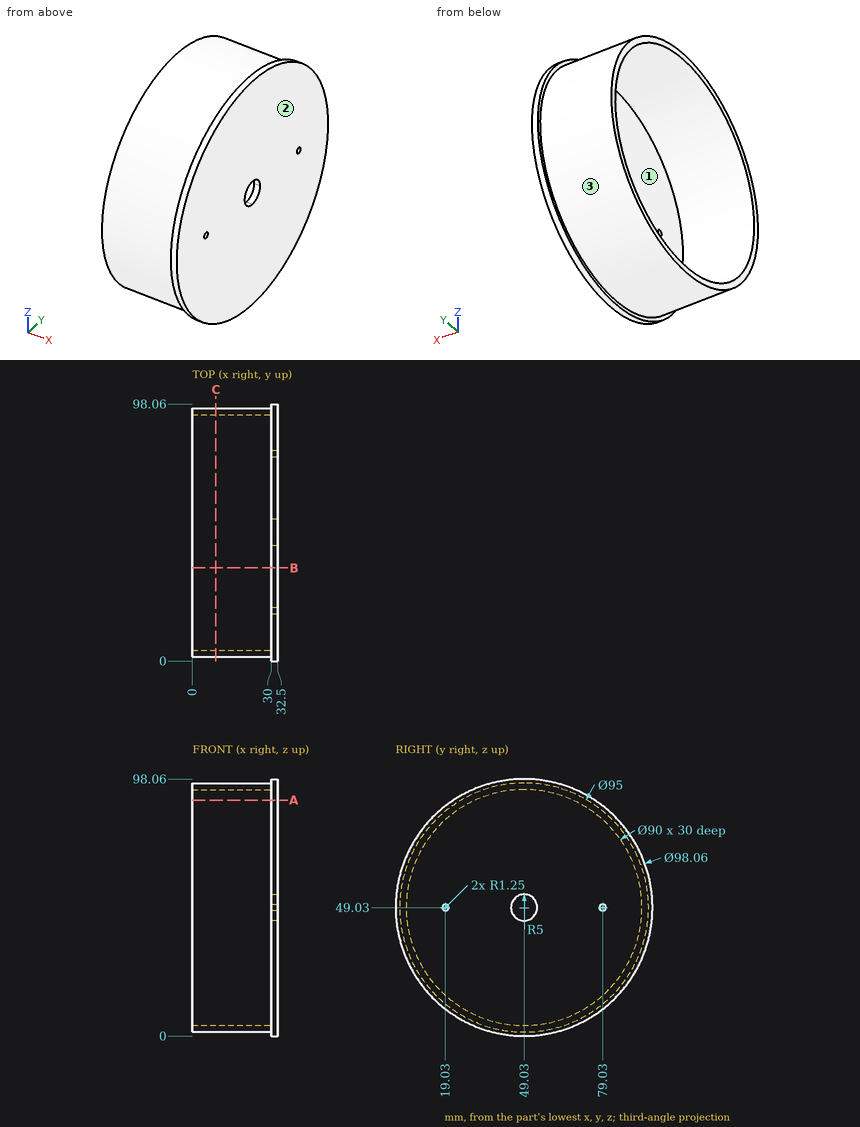
Check sheet for the drawn part. Datum: minimum x, y, z corner. Units: mm. Round coordinates to 2 decimals unless told otherwise and drop trailing zeros. Order: outer loops, then holes, each group sorted by start corner. A loop starts at its lowest first (then second) coordinate and runs counter-clockwise, first axis right, second up. Notation, with made-up numbers: (74.5, 32.5) -> (130.5, 32.5) arc R34 ccw to (130.5, 65.5) -> close; hole circle Ø4 at (61, 42.5). An arc over 180 degrees is marked (long way). Return JSON: item names as keys, results as strings. Group by question number.
Q1. Section check A-A, the plane z = 90. Record the boundary of the cut face in (x, y).
Q2. Section check B-B, the plane y = 35.5. Record the boundary of the cut face in (x, z), plus the area to 4 significant figures.
Q3. Material ranges on probe 1 along Y at (x, z) = (16.25, 49.03); probe 2 along X at (y, z) = (65, 83.5); probe 3 along Y at (x, z) = (22, 82.5), recorded low to high. Write a range as from..to.
Q4. Section check C-C, the plane x = 9. Record the boundary of the cut face in (y, z).
Q5. Gauge pin test, flat ends, axial feed: pin 1 (1 mm diameter, centred on y = 10.5, z = 18.5, fed in from -X); pin 2 (12 mm diameter, centred on x = 5, z = 76.5, fed in from -Y); pin 3 (3 mm diameter, centred on x = 19.5, z = 46.5, fed in from -Y). Record the tip position at first contact, or that the pin passes through.
Q6. Release check for a two-part mould opening along Y. For the marked faces 1, 2 and 3 record: released by +Y, released by -Y, zero draft, split by the parting line, or undercut.
Numbers:
{
 "1": {"outline": "(0, 24.99) -> (30, 24.99) -> (30, 22.1) -> (32.5, 22.1) -> (32.5, 75.96) -> (30, 75.96) -> (30, 73.07) -> (0, 73.07) -> (0, 67.64) -> (30, 67.64) -> (30, 30.42) -> (0, 30.42) -> close"},
 "2": {"outline": "(0, 3.5) -> (30, 3.5) -> (30, 1.9) -> (32.5, 1.9) -> (32.5, 96.16) -> (30, 96.16) -> (30, 94.56) -> (0, 94.56) -> (0, 91.95) -> (30, 91.95) -> (30, 6.11) -> (0, 6.11) -> close", "area": "392.5 mm^2"},
 "3": {"probe 1": "1.53..4.03, 94.03..96.53", "probe 2": "30..32.5", "probe 3": "15.33..18.95, 79.11..82.73"},
 "4": {"outline": "circle Ø95 at (49.03, 49.03); hole circle Ø90 at (49.03, 49.03)"},
 "5": {"pin 1": "x = 30", "pin 2": "y = 6.66", "pin 3": "y = 1.54"},
 "6": {"face 1": "undercut", "face 2": "zero draft", "face 3": "split by the parting line"}
}
